Could you check a few things on this model? Use its own coordinates, in mm. Face numbers are marked on the shaded views. A direction names the side the tool comes from. Round coordinates to 2 decimals unless told otherwise and drop trailing zeros. Order: outer loops, then holes, each group sorted by start corner. A loop starts at its lowest first (then second) coordinate and runs counter-clockwise, first axis right, second up. Notation, with made-up numbers: (70.5, 8.25) - (120.5, 8.25) arc R6 cw to (120.5, 19.25) - close; hole circle Ø2 at (3, 63.5). An arc over 180 degrees is marked (long way). Use one line per item in the form item = value.
from build123d import *

# Parameters (mm, degrees)
SKETCH_1_W          = 60
SKETCH_1_H          = 20
EXTRUDE_1_DEPTH     = 3
EXTRUDE_3_DEPTH     = 7
SKETCH_5_W          = 2
SKETCH_5_H          = 0.1
SKETCH_5_W_2        = 4.2
SKETCH_5_H_2        = 2
CUT_EXTRUDE_2_DEPTH = 7
CHAMFER_1_SIZE      = 0.15
FILLET_1_R          = 3


# Some blends are built 0.0001 mm under size
with BuildPart() as part:
    # 草图1 → 凸台-拉伸1 (new body)
    with BuildSketch(Plane.XY):
        with Locations((-20, 0)):
            Rectangle(SKETCH_1_W, SKETCH_1_H)
    extrude(amount=EXTRUDE_1_DEPTH)

    # 草图1<5> → 凸台-拉伸3 (add)
    with BuildSketch(Plane.XY):
        Polygon((-17.025, 10), (-23.025, 10), (-23.025, 8), (-25.025, 8), (-25.025, 6.5), (-24.525, 6), (-15.525, 6), (-15.025, 6.5), (-15.025, 8), (-17.025, 8), align=None)
        Polygon((-37.05, 10), (-43.05, 10), (-43.05, 8), (-45.05, 8), (-45.05, 6.5), (-44.55, 6), (-35.55, 6), (-35.05, 6.5), (-35.05, 8), (-37.05, 8), align=None)
        Polygon((-26, 4.55), (-26, -4.45), (-26.5, -4.95), (-28, -4.95), (-28, -2.95), (-32, -2.95), (-32, -4.95), (-33.5, -4.95), (-34, -4.45), (-34, 4.55), (-33.5, 5.05), (-32, 5.05), (-32, 3.05), (-28, 3.05), (-28, 5.05), (-26.5, 5.05), align=None)
        Polygon((-23.025, -8), (-23.025, -10), (-17.025, -10), (-17.025, -8), (-15.025, -8), (-15.025, -6.5), (-15.525, -6), (-24.525, -6), (-25.025, -6.5), (-25.025, -8), align=None)
        Polygon((-42.95, -8), (-42.95, -10), (-36.95, -10), (-36.95, -8), (-34.95, -8), (-34.95, -6.5), (-35.45, -6), (-44.45, -6), (-44.95, -6.5), (-44.95, -8), align=None)
    extrude(amount=-EXTRUDE_3_DEPTH)

    # 草图5 → 切除-拉伸2 (cut)
    with BuildSketch(Plane(origin=(0, 0, -7), x_dir=(-1, 0, 0), z_dir=(0, 0, -1))):
        with Locations((16.025, 7.95)):
            Rectangle(SKETCH_5_W, SKETCH_5_H)
        with Locations((24.025, 7.95)):
            Rectangle(SKETCH_5_W, SKETCH_5_H)
        with Locations((35.975, 7.95)):
            Rectangle(SKETCH_5_W, SKETCH_5_H)
        with Locations((43.975, 7.95)):
            Rectangle(SKETCH_5_W, SKETCH_5_H)
        with Locations((30, 4.05)):
            Rectangle(SKETCH_5_W_2, SKETCH_5_H_2)
        with Locations((30, -4.05)):
            Rectangle(SKETCH_5_W_2, SKETCH_5_H_2)
    extrude(amount=-CUT_EXTRUDE_2_DEPTH, mode=Mode.SUBTRACT)

    # 倒角1
    # the kernel refuses this chamfer: 0.15 mm, written as the material it adds along each edge
    with BuildSketch(Plane(origin=(-32.1, -3.05, -7), x_dir=(-0.027495876610573042, -0.9996219169112971, 0), z_dir=(0, 0, 1))) as chamfer_1_piece_1_section:
        Polygon((CHAMFER_1_SIZE * 0.999621916911, CHAMFER_1_SIZE * 0.0274958766106), (-CHAMFER_1_SIZE * 0.0274958766106, CHAMFER_1_SIZE * 0.999621916911), (0, 0), align=None)
    chamfer_1_piece_1 = extrude(amount=7, mode=Mode.PRIVATE)
    chamfer_1_piece_1 = split(chamfer_1_piece_1, bisect_by=Plane(origin=(-32, -3.10460455, -3.5), z_dir=(-1, 0, 0)), keep=Keep.TOP, mode=Mode.PRIVATE)
    add(chamfer_1_piece_1)
    with BuildSketch(Plane(origin=(-32.1, -3.05, -7), x_dir=(-0.027495876610573042, -0.9996219169112971, 0), z_dir=(0, 0, 1))) as chamfer_1_piece_2_section:
        Polygon((CHAMFER_1_SIZE * 0.999621916911, CHAMFER_1_SIZE * 0.0274958766106), (-CHAMFER_1_SIZE * 0.0274958766106, CHAMFER_1_SIZE * 0.999621916911), (0, 0), align=None)
    chamfer_1_piece_2 = extrude(amount=7.385752448, mode=Mode.PRIVATE)
    chamfer_1_piece_2 = split(chamfer_1_piece_2, bisect_by=Plane(origin=(-32.060343707, -3.10460455, 0), z_dir=(0, 0, 1)), keep=Keep.TOP, mode=Mode.PRIVATE)
    chamfer_1_piece_2 = split(chamfer_1_piece_2, bisect_by=Plane(origin=(-32, -3.10460455, 0.192876224), z_dir=(-1, 0, 0)), keep=Keep.TOP, mode=Mode.PRIVATE)
    add(chamfer_1_piece_2)
    with BuildSketch(Plane(origin=(-32.1, -3.05, -7), x_dir=(-0.027495876610573042, -0.9996219169112971, 0), z_dir=(0, 0, 1))) as chamfer_1_piece_3_section:
        Polygon((CHAMFER_1_SIZE * 0.999621916911, CHAMFER_1_SIZE * 0.0274958766106), (-CHAMFER_1_SIZE * 0.0274958766106, CHAMFER_1_SIZE * 0.999621916911), (0, 0), align=None)
    chamfer_1_piece_3 = extrude(amount=7.385752448, mode=Mode.PRIVATE)
    chamfer_1_piece_3 = split(chamfer_1_piece_3, bisect_by=Plane(origin=(-31.98101474, -3.063087711, 0), z_dir=(0, 0, 1)), keep=Keep.TOP, mode=Mode.PRIVATE)
    chamfer_1_piece_3 = split(chamfer_1_piece_3, bisect_by=Plane(origin=(-32, -3.063087711, 0.192876224), z_dir=(1, 0, 0)), keep=Keep.TOP, mode=Mode.PRIVATE)
    add(chamfer_1_piece_3)
    with BuildSketch(Plane(origin=(-27.9, -3.05, -7), x_dir=(-0.9996219169112968, 0.027495876610587344, 0), z_dir=(0, 0, 1))) as chamfer_1_piece_4_section:
        Polygon((CHAMFER_1_SIZE * 0.999621916911, CHAMFER_1_SIZE * 0.0274958766106), (-CHAMFER_1_SIZE * 0.0274958766106, CHAMFER_1_SIZE * 0.999621916911), (0, 0), align=None)
    chamfer_1_piece_4 = extrude(amount=7, mode=Mode.PRIVATE)
    chamfer_1_piece_4 = split(chamfer_1_piece_4, bisect_by=Plane(origin=(-28, -3.10460455, -3.5), z_dir=(1, 0, 0)), keep=Keep.TOP, mode=Mode.PRIVATE)
    add(chamfer_1_piece_4)
    with BuildSketch(Plane(origin=(-27.9, -3.05, -7), x_dir=(-0.9996219169112968, 0.027495876610587344, 0), z_dir=(0, 0, 1))) as chamfer_1_piece_5_section:
        Polygon((CHAMFER_1_SIZE * 0.999621916911, CHAMFER_1_SIZE * 0.0274958766106), (-CHAMFER_1_SIZE * 0.0274958766106, CHAMFER_1_SIZE * 0.999621916911), (0, 0), align=None)
    chamfer_1_piece_5 = extrude(amount=7.385752448, mode=Mode.PRIVATE)
    chamfer_1_piece_5 = split(chamfer_1_piece_5, bisect_by=Plane(origin=(-28.01898526, -3.063087711, 0), z_dir=(0, 0, 1)), keep=Keep.TOP, mode=Mode.PRIVATE)
    chamfer_1_piece_5 = split(chamfer_1_piece_5, bisect_by=Plane(origin=(-28, -3.063087711, 0.192876224), z_dir=(-1, 0, 0)), keep=Keep.TOP, mode=Mode.PRIVATE)
    add(chamfer_1_piece_5)
    with BuildSketch(Plane(origin=(-27.9, -3.05, -7), x_dir=(-0.9996219169112968, 0.027495876610587344, 0), z_dir=(0, 0, 1))) as chamfer_1_piece_6_section:
        Polygon((CHAMFER_1_SIZE * 0.999621916911, CHAMFER_1_SIZE * 0.0274958766106), (-CHAMFER_1_SIZE * 0.0274958766106, CHAMFER_1_SIZE * 0.999621916911), (0, 0), align=None)
    chamfer_1_piece_6 = extrude(amount=7.385752448, mode=Mode.PRIVATE)
    chamfer_1_piece_6 = split(chamfer_1_piece_6, bisect_by=Plane(origin=(-27.939656293, -3.10460455, 0), z_dir=(0, 0, 1)), keep=Keep.TOP, mode=Mode.PRIVATE)
    chamfer_1_piece_6 = split(chamfer_1_piece_6, bisect_by=Plane(origin=(-28, -3.10460455, 0.192876224), z_dir=(1, 0, 0)), keep=Keep.TOP, mode=Mode.PRIVATE)
    add(chamfer_1_piece_6)
    with BuildSketch(Plane(origin=(-32.1, 3.05, -7), x_dir=(0.9996219169112968, -0.027495876610587344, 0), z_dir=(0, 0, 1)), Plane(origin=(-27.9, 3.05, -7), x_dir=(0.02749587661059597, 0.9996219169112964, 0), z_dir=(0, 0, 1)), Plane(origin=(-42.975, 7.9, -7), x_dir=(0.027495876610572963, 0.9996219169112971, 0), z_dir=(0, 0, 1)), Plane(origin=(-23.025, 7.9, -7), x_dir=(0.02749587661059597, 0.9996219169112964, 0), z_dir=(0, 0, 1)), Plane(origin=(-17.025, 7.9, -7), x_dir=(0.9996219169112968, -0.027495876610584464, 0), z_dir=(0, 0, 1))) as chamfer_1_piece_7:
        Polygon((CHAMFER_1_SIZE * 0.999621916911, CHAMFER_1_SIZE * 0.0274958766106), (-CHAMFER_1_SIZE * 0.0274958766106, CHAMFER_1_SIZE * 0.999621916911), (0, 0), align=None)
    extrude(amount=7.385752448)
    with BuildSketch(Plane(origin=(-36.975, 7.9, -7), x_dir=(0.9996219169112968, -0.0274958766105851, 0), z_dir=(0, 0, 1))) as chamfer_1_piece_8_section:
        Polygon((CHAMFER_1_SIZE * 0.999621916911, CHAMFER_1_SIZE * 0.0274958766106), (-CHAMFER_1_SIZE * 0.0274958766106, CHAMFER_1_SIZE * 0.999621916911), (0, 0), align=None)
    chamfer_1_piece_8 = extrude(amount=7, mode=Mode.PRIVATE)
    chamfer_1_piece_8 = split(chamfer_1_piece_8, bisect_by=Plane(origin=(-36.92039545, 8, -3.5), z_dir=(0, -1, 0)), keep=Keep.TOP, mode=Mode.PRIVATE)
    add(chamfer_1_piece_8)
    with BuildSketch(Plane(origin=(-36.975, 7.9, -7), x_dir=(0.9996219169112968, -0.0274958766105851, 0), z_dir=(0, 0, 1))) as chamfer_1_piece_9_section:
        Polygon((CHAMFER_1_SIZE * 0.999621916911, CHAMFER_1_SIZE * 0.0274958766106), (-CHAMFER_1_SIZE * 0.0274958766106, CHAMFER_1_SIZE * 0.999621916911), (0, 0), align=None)
    chamfer_1_piece_9 = extrude(amount=7.385752448, mode=Mode.PRIVATE)
    chamfer_1_piece_9 = split(chamfer_1_piece_9, bisect_by=Plane(origin=(-36.92039545, 7.939656293, 0), z_dir=(0, 0, 1)), keep=Keep.TOP, mode=Mode.PRIVATE)
    chamfer_1_piece_9 = split(chamfer_1_piece_9, bisect_by=Plane(origin=(-36.92039545, 8, 0.192876224), z_dir=(0, -1, 0)), keep=Keep.TOP, mode=Mode.PRIVATE)
    add(chamfer_1_piece_9)
    with BuildSketch(Plane(origin=(-36.975, 7.9, -7), x_dir=(0.9996219169112968, -0.0274958766105851, 0), z_dir=(0, 0, 1))) as chamfer_1_piece_10_section:
        Polygon((CHAMFER_1_SIZE * 0.999621916911, CHAMFER_1_SIZE * 0.0274958766106), (-CHAMFER_1_SIZE * 0.0274958766106, CHAMFER_1_SIZE * 0.999621916911), (0, 0), align=None)
    chamfer_1_piece_10 = extrude(amount=7.385752448, mode=Mode.PRIVATE)
    chamfer_1_piece_10 = split(chamfer_1_piece_10, bisect_by=Plane(origin=(-36.961912289, 8.01898526, 0), z_dir=(0, 0, 1)), keep=Keep.TOP, mode=Mode.PRIVATE)
    chamfer_1_piece_10 = split(chamfer_1_piece_10, bisect_by=Plane(origin=(-36.961912289, 8, 0.192876224), z_dir=(0, 1, 0)), keep=Keep.TOP, mode=Mode.PRIVATE)
    add(chamfer_1_piece_10)
    with BuildSketch(Plane(origin=(-36.95, -8, 0.385752448), x_dir=(-0.027495876610572963, -0.9996219169112971, 0), z_dir=(0, 0, -1)), Plane(origin=(-42.95, -8, 0.385752448), x_dir=(-0.9996219169112968, 0.0274958766105851, 0), z_dir=(0, 0, -1)), Plane(origin=(-17.025, -8, 0.385752448), x_dir=(-0.02749587661059597, -0.9996219169112964, 0), z_dir=(0, 0, -1)), Plane(origin=(-23.025, -8, 0.385752448), x_dir=(-0.9996219169112968, 0.027495876610584464, 0), z_dir=(0, 0, -1))) as chamfer_1_piece_11:
        Polygon((CHAMFER_1_SIZE * 0.999621916911, -CHAMFER_1_SIZE * 0.0274958766106), (-CHAMFER_1_SIZE * 0.0274958766106, -CHAMFER_1_SIZE * 0.999621916911), (0, 0), align=None)
    extrude(amount=7.385752448)
    # the kernel refuses this chamfer: 0.15 mm, written as the material it takes off along each edge
    with BuildSketch(Plane(origin=(-32.1, -4.95, -7.385752448), x_dir=(-0.9996219169112968, -0.0274958766105851, 0), z_dir=(0, 0, 1)), Plane(origin=(-32.1, 5.05, -7.385752448), x_dir=(0.027495876610572963, -0.9996219169112971, 0), z_dir=(0, 0, 1)), Plane(origin=(-27.9, 5.05, -7.385752448), x_dir=(0.9996219169112968, 0.027495876610584464, 0), z_dir=(0, 0, 1)), Plane(origin=(-25.025, 7.9, -7.385752448), x_dir=(0.9996219169112968, 0.027495876610584464, 0), z_dir=(0, 0, 1)), Plane(origin=(-35.05, 7.9, -7.385752448), x_dir=(0.027495876610572963, -0.9996219169112971, 0), z_dir=(0, 0, 1)), Plane(origin=(-15.025, 7.9, -7.385752448), x_dir=(0.027495876610584464, -0.9996219169112968, 0), z_dir=(0, 0, 1))) as chamfer_1_2_piece_1:
        Polygon((CHAMFER_1_SIZE * 0.999621916911, -CHAMFER_1_SIZE * 0.0274958766106), (-CHAMFER_1_SIZE * 0.0274958766106, -CHAMFER_1_SIZE * 0.999621916911), (0, 0), align=None)
    extrude(amount=7.385752448, mode=Mode.SUBTRACT)
    with BuildSketch(Plane(origin=(-27.9, -4.95, 0), x_dir=(-0.02749587661059597, 0.9996219169112964, 0), z_dir=(0, 0, -1)), Plane(origin=(-34.95, -8, 0), x_dir=(-0.9996219169112968, -0.0274958766105851, 0), z_dir=(0, 0, -1)), Plane(origin=(-44.95, -8, 0), x_dir=(-0.027495876610572963, 0.9996219169112971, 0), z_dir=(0, 0, -1)), Plane(origin=(-15.025, -8, 0), x_dir=(-0.9996219169112968, -0.027495876610584464, 0), z_dir=(0, 0, -1)), Plane(origin=(-25.025, -8, 0), x_dir=(-0.02749587661059597, 0.9996219169112964, 0), z_dir=(0, 0, -1))) as chamfer_1_2_piece_2:
        Polygon((CHAMFER_1_SIZE * 0.999621916911, CHAMFER_1_SIZE * 0.0274958766106), (-CHAMFER_1_SIZE * 0.0274958766106, CHAMFER_1_SIZE * 0.999621916911), (0, 0), align=None)
    extrude(amount=7.385752448, mode=Mode.SUBTRACT)

    # 圆角1
    fillet_1_edges = [part.edges().sort_by_distance(p)[0] for p in [
        (10, 0, 3),
        (-20, -10, 3),
        (-20, 10, 3),
        (-50, 0, 3),
    ]]
    fillet(fillet_1_edges, radius=FILLET_1_R - 0.0001)  # a hair under: the kernel refuses the full size


solid = part.part
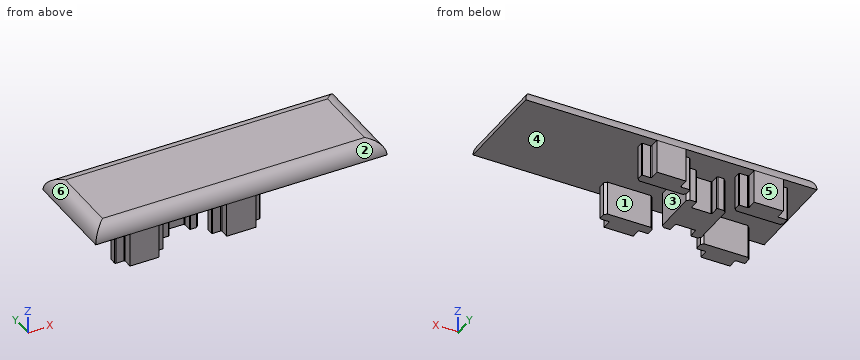
Item 1: For the marked faces 1, 2 and 3, which set-ups out of +Z, -Z, +X, -X, +Y, -Y let a thin tool reach every point of the face, with its end or its side?
Found:
face_1 = -Z, +X, -X
face_2 = +Z, +X, -X, -Y
face_3 = -Z, +X, +Y, -Y
Item 2: If we mould it in two halves opening along Y, with no side actions, what happens to the marked faces 4, 5 and 6? For each: released by +Y, released by -Y, zero draft, split by the parting line, or undercut.
Found:
face_4 = undercut
face_5 = released by +Y
face_6 = zero draft
Item 3: Will these pins go through, and if not, where does the flat tip stop? P1, Ø0.8, axis at x = -36, z = -5, coming from the +Y side; P2, Ø6, axis at y = 7.5, z = -3.5, coming from the +X side (3 decimals); P3, Ø1.8, axis at y = -3.5, z = -4, coming from the +X side.
Found:
P1 = 7.9
P2 = -15.025
P3 = -26
Item 4: Imagine slicing it at A-A on x = -40.5. Please give me the cut outline in (y, z).
Found:
outline = (-10, -7) - (-6, -7) - (-6, 0) - (6, 0) - (6, -7) - (10, -7) - (10, 0) arc R3 ccw to (7, 3) - (-7, 3) arc R3 ccw to (-10, 0) - close
Item 5: I need wall thicknesses on L1, parallel to Y at x = -23.5, z = -0.75; L2, parallel to Y at x = -22.5, z = -2.75; L3, parallel to X at y = -3, z = -3. Which ranges of each line are inside material? Lowest first, please.
Found:
L1 = -8 to -6, 6 to 7.9
L2 = -10 to -6, 6 to 10
L3 = -34 to -32, -28 to -26
Item 6: Imagine slicing it at C-C on z = -2.25. State how many separate pieces and enclosed holes the cut face has, plus the area to 3 significant figures.
Found:
separate_pieces = 5
enclosed_holes = 0
area = 189 mm2
